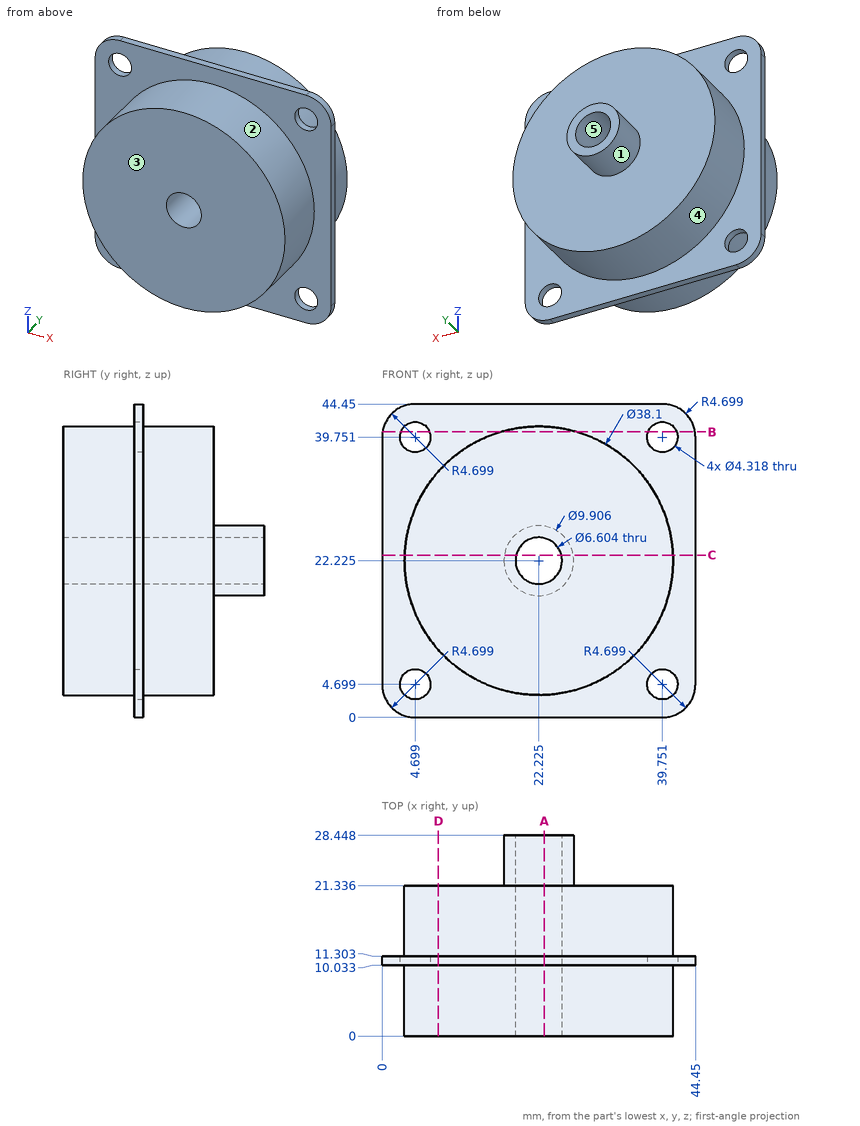
Print and shaded views of the part. All mm, measured from the part's lowest x, y and z. A direction names the side the tool comes from. Coordinates: 2 decimals unless noted, no trailing zeros. Order: outer loops, then holes, each group sorted by start corner. A loop starts at its lowest first (then second) coordinate and runs counter-clockwise, first axis right, second up. Notation, with made-up numbers: (44.25, 65.25) - (52.25, 65.25) arc R8 ccw to (52.25, 71.25) - close; hole circle Ø6 at (14.25, 73). An arc over 180 degrees is marked (long way). Return JSON: item names as keys, results as strings. Group by question number.
Item 1: Drill centre lines: probe 1 along Z at (x, y) = (22.5, 16.5); probe 2 along Y at (x, z) = (12, 28.5); probe 3 along Y at (x, z) = (42.5, 11). Where is each one in solid material? Low to high. Write a range as from..to.
Item 2: Cut at D-D (x = 8). List the corners of the cut face in (y, z).
Item 3: Cut at C-C (z = 23). List the corners of the cut face in (x, y), plus the area to 3 significant figures.
Item 4: Pull direction Z, two halves, no side cores. Call the marked faces 3, 4 and 5: pulls with the +Z half, pulls with the -Z half, needs draft (parallel to the pull), parting line crosses it, or undercut.
Item 5: Which spindle directions (+Z, -Z, +X, -X, +Y, -Y) get a long thin tool onto all of the face, cutting with end or side? Do the marked faces 1 and 2. Say none if no direction does.
Item 6: Cut at A-A (x = 23). List the corners of the cut face in (y, z).
Item 7: Cut at B-B (z = 40.5). List the corners of the cut face in (x, y).
Item 8: Pin check, flat tips, straight feed: pin 1 (6 mm diameter, centred on x = 29.5, y = 17.5, fed in from -Z); pin 2 (5.5 mm diameter, centred on x = 4.699, z = 4.699, fed in from -Y); pin 3 (4 mm diameter, centred on x = 39.751, z = 4.699, fed in from +Y); pin 4 (3 mm diameter, centred on x = 19, z = 31.5, fed in from +Y). Stop position of each tip, or through.
Check values:
{
 "1": {"probe 1": "z = 3.18..18.93, 25.52..41.27", "probe 2": "y = 0..21.34", "probe 3": "y = 10.03..11.3"},
 "2": {"outline": "(0, 9.55) - (10.03, 9.55) - (10.03, 0) - (11.3, 0) - (11.3, 9.55) - (21.34, 9.55) - (21.34, 34.9) - (11.3, 34.9) - (11.3, 44.45) - (10.03, 44.45) - (10.03, 34.9) - (0, 34.9) - close"},
 "3": {"outline": "(0, 10.03) - (3.19, 10.03) - (3.19, 0) - (19.02, 0) - (19.02, 28.45) - (17.33, 28.45) - (17.33, 21.34) - (3.19, 21.34) - (3.19, 11.3) - (0, 11.3) - close; (25.43, 0) - (41.26, 0) - (41.26, 10.03) - (44.45, 10.03) - (44.45, 11.3) - (41.26, 11.3) - (41.26, 21.34) - (27.12, 21.34) - (27.12, 28.45) - (25.43, 28.45) - close", "area": "707 mm2"},
 "4": {"face 3": "needs draft", "face 4": "parting line crosses it", "face 5": "undercut"},
 "5": {"face 1": "+Y", "face 2": "-Y"},
 "6": {"outline": "(0, 3.19) - (10.03, 3.19) - (10.03, 0) - (11.3, 0) - (11.3, 3.19) - (21.34, 3.19) - (21.34, 17.33) - (28.45, 17.33) - (28.45, 19.02) - (0, 19.02) - close; (0, 25.43) - (28.45, 25.43) - (28.45, 27.12) - (21.34, 27.12) - (21.34, 41.26) - (11.3, 41.26) - (11.3, 44.45) - (10.03, 44.45) - (10.03, 41.26) - (0, 41.26) - close"},
 "7": {"outline": "(0.06, 10.03) - (2.67, 10.03) - (2.67, 11.3) - (0.06, 11.3) - close; (6.72, 10.03) - (16.85, 10.03) - (16.85, 0) - (27.6, 0) - (27.6, 10.03) - (37.73, 10.03) - (37.73, 11.3) - (27.6, 11.3) - (27.6, 21.34) - (16.85, 21.34) - (16.85, 11.3) - (6.72, 11.3) - close; (41.78, 10.03) - (44.39, 10.03) - (44.39, 11.3) - (41.78, 11.3) - close"},
 "8": {"pin 1": "stops at z = 3.66", "pin 2": "stops at y = 10.03", "pin 3": "passes through", "pin 4": "stops at y = 21.34"}
}
